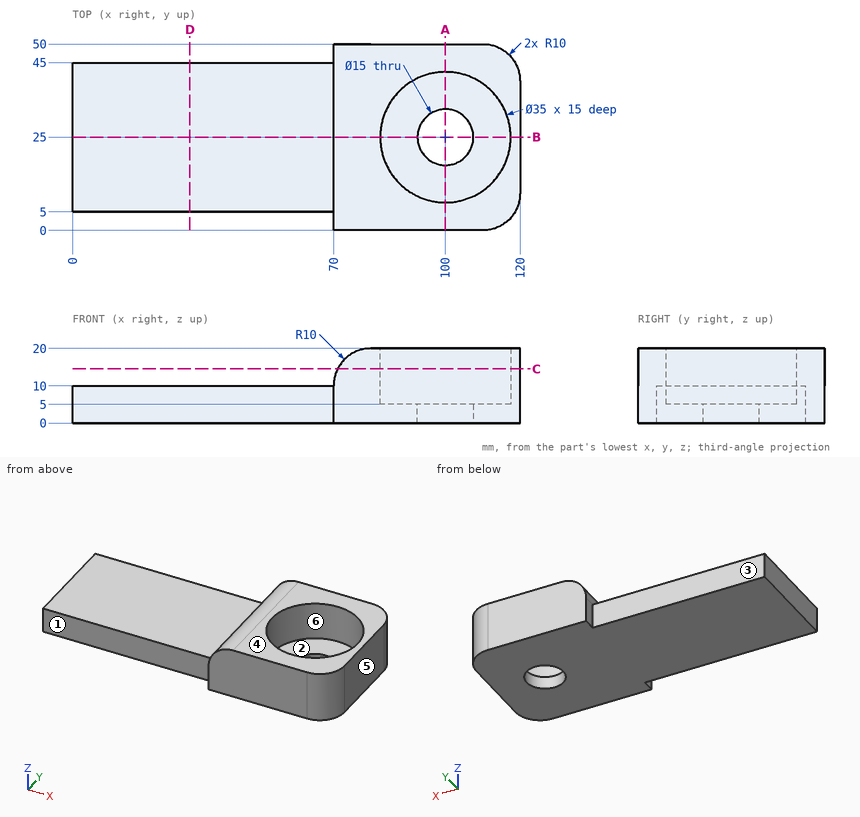
Source: three-view drawing plus pictorial views. Frame: mm from the lowest corner of the part. A direction names the side the tool comes from. Round coordinates to 2 decimals unless told otherwise and drop trailing zeros. Write each loop counter-clockwise with the first axis right and the second up, starting at its lowest first coordinate (ties: lowest second). Pieces come first, ordered by that corner, then holes. Notation, with made-up numbers: M 64.5,79 L 100.5,79 A33 cw 100.5,113 Z; hole C 2,77.25 d6. An arc over 180 degrees is marked long. One line per item, written item: value. Start each with the question number.
Item 1: Set-up query: the marked faces 1, 2 and 3. Return all of +Z, -Z, +X, -X, +Y, -Y with unobstructed straight access to the full face (end or side cutting, diameter ignored); none if empty.
Item 2: Mould query, pull axis X, two halves, no side actions, for the marked faces 4, 5 and 6. Classes: pulls with the +X half, pulls with the -X half, needs draft (parallel to the pull), parting line crosses it, or undercut.
Item 3: Section query D-D (x = 31.5). Return the cut outline in (y, z).
Item 4: Section query A-A (x = 100). Return the cut outline in (y, z).
Item 5: Section query C-C (z = 14.5). Return the cut outline in (x, y).
Item 6: Pin query (flat end, axial travel): pin 1 (24 mm diameter, centred on x = 100, y = 25, fed in from +Z); pin 2 (6 mm diameter, centred on y = 11, z = 4, fed in from -X); pin 3 (8 mm diameter, centred on x = 65.5, z = 4, fed in from -Y); pin 4 (1 mm diameter, centred on x = 47, z = 8.5, fed in from +Y). Return the tip coordinate at first contact, or that it passes through.
Item 7: Ray query, L1, parallel to Z at x = 37.5, y = 41.5; L2, parallel to Y at x = 100, z = 2.55; L3, parallel to X at y = 33, z = 5.5. Return the intervals inside material, ascending. Write a range as from..to.
Item 8: Section query B-B (y = 25). Return the cut outline in (x, z), plus the area to 3 significant figures.
Result set:
1. face 1: +Z, -Z, -X, -Y
1. face 2: +Z
1. face 3: +Z, -Z, -X, +Y
2. face 4: needs draft
2. face 5: pulls with the +X half
2. face 6: undercut
3. outline: M 5,0 L 45,0 L 45,10 L 5,10 Z
4. outline: M 0,0 L 17.5,0 L 17.5,5 L 7.5,5 L 7.5,20 L 0,20 Z; M 32.5,0 L 50,0 L 50,20 L 42.5,20 L 42.5,5 L 32.5,5 Z
5. outline: M 71.07,0 L 110,0 A10 ccw 120,10 L 120,40 A10 ccw 110,50 L 71.07,50 Z; hole C 100,25 d35
6. pin 1: stops at z = 5
6. pin 2: stops at x = 0
6. pin 3: stops at y = 5
6. pin 4: stops at y = 45
7. L1: z = 0..10
7. L2: y = 0..17.5, 32.5..50
7. L3: x = 0..84.44, 115.56..120
8. outline: M 0,0 L 92.5,0 L 92.5,5 L 82.5,5 L 82.5,20 L 80,20 A10 ccw 70,10 L 0,10 Z; M 107.5,0 L 120,0 L 120,20 L 117.5,20 L 117.5,5 L 107.5,5 Z
8. area: 1,080 mm²
